Design review of the part shown in the three views and the two pictorial views. Dimensions are in mm from the part's minimum x, y and z. Round coordinates to 2 decimals unless told otherwise and drop trailing zeros. Loops run counter-clockwise (first coordinate to the right, second up) from the corner with the lowest first, then second, coordinate; pieces in that order, holes last. Notation, with made-up numbers: (27.5, -18.5) -> (45.5, -18.5) arc R10 cw to (45.5, -12.5) -> close; hole circle Ø3 at (-29.75, 80.5). An arc over 180 degrees is marked (long way). Return JSON: item names as keys, results as strings. Group by question number.
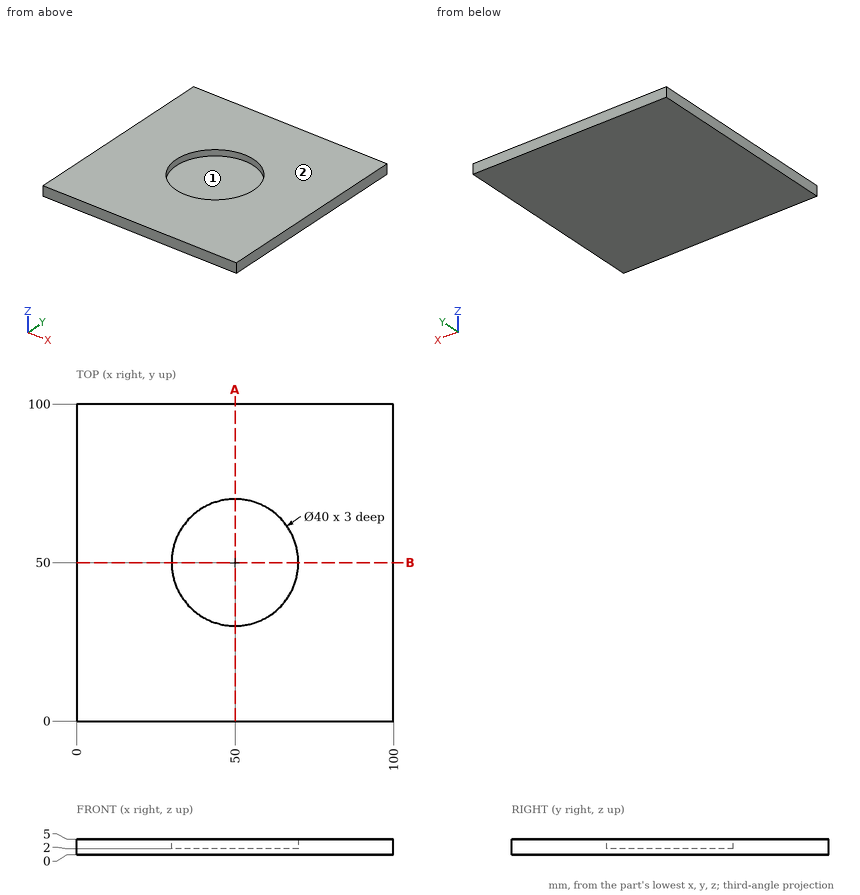
1. We need section A-A, the plane x = 50. Write out the cut boundary in (y, z), then the cut area to 3 significant figures.
2. Wall thickness on line 1 (Y direction, x = 50, z = 4.15); line 2 (Z direction, x = 59.5, y = 55.5); line 3 (Y direction, x = 52.5, z = 4.6): over which ranges is each line inside the solid? List them lowest first.
3. For P1, Ø10, axis at x = 40.5, y = 57.5, coming from the +Z side; P2, Ø3, axis at y = 37, z = 1, coming from the -X side, all flat-tipped, find the tip position at first contact; note any pin that passes through.
4. Draft analysis for pull direction Y (two halves, no side actions). For the marked faces 1 and 2, state which applies: pulls with the +Y half, pulls with the -Y half, needs draft (parallel to the pull), parting line crosses it, or undercut.
Check sheet entries:
{
 "1": {"outline": "(0, 0) -> (100, 0) -> (100, 5) -> (70, 5) -> (70, 2) -> (30, 2) -> (30, 5) -> (0, 5) -> close", "area": "380 mm²"},
 "2": {"line 1": "y = 0 to 30, 70 to 100", "line 2": "z = 0 to 2", "line 3": "y = 0 to 30.16, 69.84 to 100"},
 "3": {"P1": "stops at z = 2", "P2": "stops at x = 0"},
 "4": {"face 1": "undercut", "face 2": "needs draft"}
}
